Read the model definition and answer for the solid it produces. Units are mm, in the model's axes. Face numbers are marked on the shaded views. A direction names the side the tool comes from. Coordinates: 2 decimals unless noted, no trailing zeros. Order: outer loops, then holes, each group sorted by start corner. A loop starts at its lowest first (then second) coordinate and runs counter-clockwise, first axis right, second up. Notation, with made-up numbers: (30, 66) -> (54, 66) arc R13 cw to (54, 78) -> close; hole circle Ø6 at (42.25, 86). An arc over 180 degrees is marked (long way). Answer as a JSON object with one key per item and string values. Group by question number.
1) Consider L1, parallel to Z at x = -1.75, y = -1.5; L2, parallel to Y at x = 0, z = 10.75; L3, parallel to X at y = 0.25, z = 9. Determine where each line is inside the solid, lowest interval first.
2) A tool of negligible diameter and unlimited length cuts with its end or side. For the marked faces 1 and 2, from which of +Z, -Z, +X, -X, +Y, -Y can it reach the whole face along a straight path? Write none if from no direction.
3) Section C-C on z = 7 is taken. Determine the outline of the cut face in (x, y), and give its area (3 significant figures).
4) Given pin 1 (1 mm diameter, centred on x = 0.5, z = 6, fed in from +Y); pin 2 (1.5 mm diameter, centred on y = 0, z = 10, fed in from +X), each flat-ended and moving along its own axis, determine where each tip first touches the part or whether it passes through.
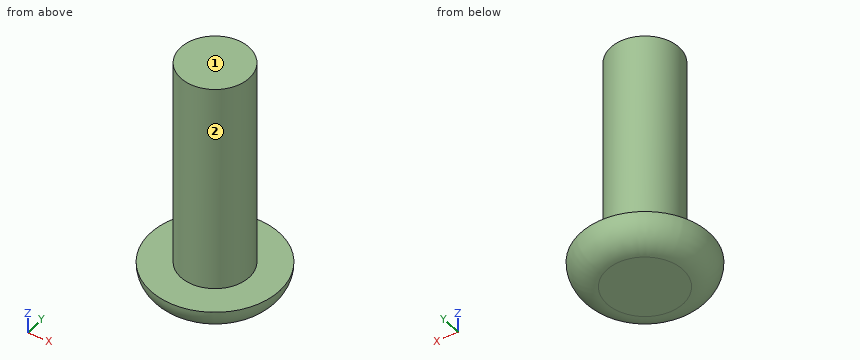
Autodesk Inventor part; units mm, degrees
ref_plane "YZ Plane" through (0, 0, 0) normal (1, 0, 0) x (0, 1, 0)
ref_plane "XZ Plane" through (0, 0, 0) normal (0, 1, 0) x (-1, 0, 0)
ref_plane "XY Plane" through (0, 0, 0) normal (0, 0, 1) x (1, 0, 0)
sketch "Sketch1" plane through (0, 0, 0) normal (0, 0, 1) x (1, 0, 0)
  circle A0 centre (0, 0) radius 3.8735
  dimension "d0" = 7.747
extrude "Extrusion1" add sketch "Sketch1" along normal blind 1.5875
fillet "Fillet1" radius 1.5875 1 edges at (-3.8735, 0, 0)
sketch "Sketch2" plane through (0, 0, 1.5875) normal (0, 0, 1) x (1, 0, 0)
  circle A0 centre (0, 0) radius 3.8735
  circle A1 centre (0, 0) radius 2.0574
  dimension "d4" = 4.1148
extrude "Extrusion2" add sketch "Sketch2" along normal blind 12.7 contours A1
thread "Thread1"
properties part number "8-32 Screw"
Worked answers:
{
 "1": {"L1": "z = 0 to 1.59", "L2": "y = -2.06 to 2.06", "L3": "x = -2.04 to 2.04"},
 "2": {"face 1": "+Z, +X, -X, +Y, -Y", "face 2": "+Z"},
 "3": {"outline": "circle Ø4.11 at (0, 0)", "area": "13.3 mm²"},
 "4": {"pin 1": "stops at y = 2.06", "pin 2": "stops at x = 2.06"}
}
